```python
from build123d import *

# Parameters (mm, degrees)
SKETCH2_R           = 53
CUT_EXTRUDE1_DEPTH  = 13
SKETCH3_R           = 5.5
CUT_EXTRUDE2_DEPTH  = 233.304143312
SKETCH4_R           = 6
CUT_EXTRUDE3_DEPTH  = 20
SKETCH5_R           = 30
BOSS_EXTRUDE1_DEPTH = 10


with BuildPart() as part:
    # Sketch1 → Revolve1 (revolve)
    with BuildSketch(Plane(origin=(0, 0, 0), x_dir=(0, 0, -1), z_dir=(1, 0, 0))):
        Polygon((-29, 0), (-99.5, 0), (-99.5, 5), (-125, 5), (-125, 17), (-125.25, 17), (-125.25, 60.6), (-125, 60.6), (-125, 72.6), (-110, 72.6), (-110, 70.1), (-107, 70.1), (-107, 72.6), (-96, 72.6), (-96, 82.5), (-40, 82.5), (-40, 103.15), (-99.75, 103.15), (-99.75, 111), (-43.5, 111), (-43.5, 112), (-40, 112), (-40, 122.3), (-32.5, 122.3), (-32.5, 155.3), (-29, 155.3), align=None)
    revolve(axis=Axis((0, 155.3, 0), (0, -1, 0)))

    # Sketch2 → Cut-Extrude1 (cut)
    with BuildSketch(Plane.XZ):
        with Locations(Location((0, 0, 0), (0, 0, 270))):
            Circle(SKETCH2_R)
    extrude(amount=-CUT_EXTRUDE1_DEPTH, mode=Mode.SUBTRACT)

    # Sketch3 → Cut-Extrude2 (cut, through all)
    with BuildSketch(Plane.XZ.offset(-5)):
        with Locations(Location((-116.5, 0, 0), (0, 0, 270))):
            Circle(SKETCH3_R)
        with Locations(Location((-107.631965538, 44.582619871, 0), (0, 0, 270))):
            Circle(SKETCH3_R)
        with Locations(Location((-82.377940008, 82.377940008, 0), (0, 0, 270))):
            Circle(SKETCH3_R)
        with Locations(Location((-44.582619871, 107.631965538, 0), (0, 0, 270))):
            Circle(SKETCH3_R)
        with Locations(Location((0, 116.5, 0), (0, 0, 270))):
            Circle(SKETCH3_R)
        with Locations(Location((44.582619871, 107.631965538, 0), (0, 0, 270))):
            Circle(SKETCH3_R)
        with Locations(Location((82.377940008, 82.377940008, 0), (0, 0, 270))):
            Circle(SKETCH3_R)
        with Locations(Location((107.631965538, 44.582619871, 0), (0, 0, 270))):
            Circle(SKETCH3_R)
        with Locations(Location((116.5, 0, 0), (0, 0, 270))):
            Circle(SKETCH3_R)
        with Locations(Location((107.631965538, -44.582619871, 0), (0, 0, 270))):
            Circle(SKETCH3_R)
        with Locations(Location((82.377940008, -82.377940008, 0), (0, 0, 270))):
            Circle(SKETCH3_R)
        with Locations(Location((0, -116.5, 0), (0, 0, 270))):
            Circle(SKETCH3_R)
        with Locations(Location((-44.582619871, -107.631965538, 0), (0, 0, 270))):
            Circle(SKETCH3_R)
        with Locations(Location((-82.377940008, -82.377940008, 0), (0, 0, 270))):
            Circle(SKETCH3_R)
    extrude(amount=-CUT_EXTRUDE2_DEPTH, mode=Mode.SUBTRACT)

    # Sketch4 → Cut-Extrude3 (cut)
    with BuildSketch(Plane(origin=(0, 0, 0), x_dir=(-1, 0, 0), z_dir=(0, -1, 0))):
        with Locations(Location((80, 0, 0), (0, 0, 90))):
            Circle(SKETCH4_R)
        with Locations(Location((69.282032303, -40, 0), (0, 0, 90))):
            Circle(SKETCH4_R)
        with Locations(Location((0, -80, 0), (0, 0, 90))):
            Circle(SKETCH4_R)
        with Locations(Location((-40, -69.282032303, 0), (0, 0, 90))):
            Circle(SKETCH4_R)
        with Locations(Location((-69.282032303, -40, 0), (0, 0, 90))):
            Circle(SKETCH4_R)
        with Locations(Location((-69.282032303, 40, 0), (0, 0, 90))):
            Circle(SKETCH4_R)
        with Locations(Location((-40, 69.282032303, 0), (0, 0, 90))):
            Circle(SKETCH4_R)
        with Locations(Location((0, 80, 0), (0, 0, 90))):
            Circle(SKETCH4_R)
        with Locations(Location((69.282032303, 40, 0), (0, 0, 90))):
            Circle(SKETCH4_R)
    extrude(amount=-CUT_EXTRUDE3_DEPTH, mode=Mode.SUBTRACT)

    # Sketch5 → Boss-Extrude1 (add)
    with BuildSketch(Plane(origin=(0, 82.5, 0), x_dir=(1, 0, 0), z_dir=(0, 1, 0))):
        with Locations(Location((0, 71, 0), (0, 0, 50.244401083))):
            Circle(SKETCH5_R)
        with Locations(Location((61.487803669, -35.5, 0), (0, 0, 9.755598917))):
            Circle(SKETCH5_R)
        with Locations(Location((-61.487803669, -35.5, 0), (0, 0, 170.244401083))):
            Circle(SKETCH5_R)
    extrude(amount=BOSS_EXTRUDE1_DEPTH)


solid = part.part
```
The model under review builds one solid part; all positions refer to its coordinate system, in mm. A direction names the side the tool comes from. Round coordinates to 2 decimals unless told otherwise and drop trailing zeros. Order: outer loops, then holes, each group sorted by start corner. A loop starts at its lowest first (then second) coordinate and runs counter-clockwise, first axis right, second up. Notation, with made-up numbers: (0, 26.5) -> (16, 26.5) arc R20 ccw to (16, 42.5) -> close; hole circle Ø2 at (-12, 42). An arc over 180 degrees is marked (long way). One line per item, written item: value. Start each with the question number.
Q1. Clearance check with flat-ended pins moving along their axes: pin 1 Ø8 at (x, z) = (-96.5, 37.5) entering from +Y; pin 2 Ø4 at (x, y) = (99.5, 59) entering from +Z; pin 3 Ø17.5 at (x, z) = (107.63, 44.58) entering from +Y. State where each tip first meets the part, or that it passes through.
Q2. Wall thickness on line 1 (X direction, y = 5.5, z = 0); line 2 (Y direction, x = 93, z = -20); line 3 (X direction, y = 38, z = 110): over which ranges is each line inside the solid? List them lowest first.
Q3. Mouldability with a two-part tool opening along Z and no side actions: class faces 1 (the face through (-84, 82.5, 49)), 2 (the face through (25.73, 83.15, 13.38)), 3 (the face through (-5.5, 66.68, -124.88)) as released by +Z, released by -Z, zero draft, split by the parting line, or undercut.
Q4. Take a section at B-B (z = 0). Count the separate pieces of the cut face and the enclosed holes in it, and give its area (3 significant figures).
Q5. Take a section at C-C (z = -116.5). Write out the cut boundary in (x, y).
Q6. Take a section at A-A (x = -116.5). Write out the cut boundary in (y, z).
Q7. Machinability: for faces 4 (the face through (63.425, 9.86, 41.301)), 5 (the face through (95, 72.6, -16)), 6 (the face through (39.05, 117.22, -8.67)), which of the approach directions +Z, -Z, +X, -X, +Y, -Y give a long, thin tool a straight path to every point of the face, cutting with its end or side? Answer none if there is none.
Reported:
1. pin 1: stops at y = 111
1. pin 2: stops at z = 78.62
1. pin 3: stops at y = 72.6
2. line 1: x = -125 to -122, -111 to -86, -74 to -53, 53 to 111, 122 to 125
2. line 2: y = 0 to 82.5, 103.15 to 111
2. line 3: x = -59.9 to -49.55, -39.62 to 39.62, 49.55 to 59.9
3. face 1: zero draft
3. face 2: undercut
3. face 3: split by the parting line
4. separate pieces: 4
4. enclosed holes: 0
4. area: 14,700 mm2
5. outline: (-45.99, 17) -> (-45.31, 17) -> (-45.31, 5) -> (-5.5, 5) -> (-5.5, 72.6) -> (-45.31, 72.6) -> (-45.31, 60.6) -> (-45.99, 60.6) -> close; (5.5, 5) -> (45.31, 5) -> (45.31, 17) -> (45.99, 17) -> (45.99, 60.6) -> (45.31, 60.6) -> (45.31, 72.6) -> (5.5, 72.6) -> close
6. outline: (5, -45.31) -> (17, -45.31) -> (17, -45.99) -> (60.6, -45.99) -> (60.6, -45.31) -> (72.6, -45.31) -> (72.6, -5.5) -> (5, -5.5) -> close; (5, 5.5) -> (72.6, 5.5) -> (72.6, 45.31) -> (60.6, 45.31) -> (60.6, 45.99) -> (17, 45.99) -> (17, 45.31) -> (5, 45.31) -> close
7. face 4: -Y
7. face 5: none
7. face 6: +Y
